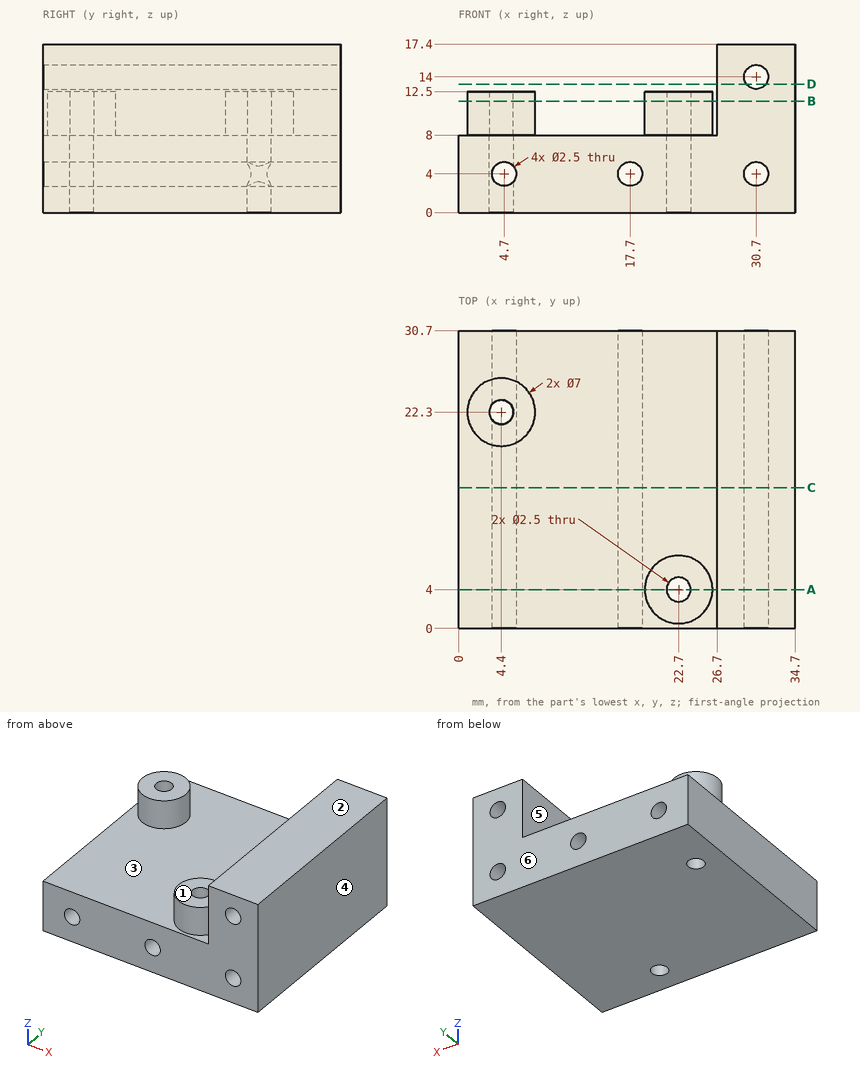
Input: dimensioned drawing with shaded views. Units: mm. Origin: part minimum x, y, z. A direction names the side the tool comes from. Round coordinates to 2 decimals unless told otherwise and drop trailing zeros. Order: outer loops, then holes, each group sorted by start corner. A loop starts at its lowest first (then second) coordinate and runs counter-clockwise, first axis right, second up. Notation, with made-up numbers: (31.25, 28) - (81.25, 28) arc R24 ccw to (81.25, 44) - close; hole circle Ø10 at (1, 70). An arc over 180 degrees is marked (long way). Use CSV: the item, a comma, the result in double quotes. Start each with the question number.
Q1. Section query B-B (z = 11.5). Return loops of the section in (x, y).
Q2. Section query A-A (y = 4). Return loops of the section in (x, z).
Q3. Material intervals for line 1 along X through (y, z) = (21.5, 12); line 2 along X through (y, z) = (13.5, 3.5); line 3 along Z through (x, y) = (19.5, 27.5), sorted ascending. Write a range as from..to.
Q4. Section query C-C (y = 14.5). Return loops of the section in (x, z).
Q5. First-contact query: pin 1 (3 mm diameter, centred on x = 17.7, z = 4, fed in from -Y); pin 2 (2 mm diameter, centred on x = 5.5, y = 22, fed in from +Z); pin 3 (1.5 mm diameter, centred on y = 5, z = 10, fed in from -X); pin 4 (1 mm diameter, centred on x = 19, y = 17, fed in from +Z). Flat tips, straight axial feed; report the tip coordinate or a pass-through.
Q6. Mould query, pull axis X, two halves, no side actions, for the marked faces 4, 5 and 6. Classes: +X half, -X half, draft (parallel to the pull), parting line (faces both ways), or undercut.
Q7. Section query D-D (z = 13.25). Return loops of the section in (x, y), and give its area (3 significant figures).
Q8. Access query for the marked faces 1, 2 and 3. Directions: +Z, -Z, +X, -X, +Y, -Y. A direction counts if a zero-diameter tool reaches every point of the face in a straight line with its end or side. Return the directions, or none.
Result set:
1,outline,"circle Ø7 at (4.4, 22.3); circle Ø7 at (22.7, 4); (26.7, 0) - (34.7, 0) - (34.7, 30.7) - (26.7, 30.7) - close; hole circle Ø2.5 at (4.4, 22.3); hole circle Ø2.5 at (22.7, 4)"
2,outline,"(0, 0) - (21.45, 0) - (21.45, 12.5) - (19.2, 12.5) - (19.2, 8) - (0, 8) - close; (23.95, 0) - (34.7, 0) - (34.7, 17.4) - (26.7, 17.4) - (26.7, 8) - (26.2, 8) - (26.2, 12.5) - (23.95, 12.5) - close; hole circle Ø2.5 at (4.7, 4); hole circle Ø2.5 at (17.7, 4); hole circle Ø2.5 at (30.7, 4); hole circle Ø2.5 at (30.7, 14)"
3,line 1,"x = 0.99..3.44, 5.36..7.81, 26.7..34.7"
3,line 2,"x = 0..3.55, 5.85..16.55, 18.85..29.55, 31.85..34.7"
3,line 3,"z = 0..8"
4,outline,"(0, 0) - (34.7, 0) - (34.7, 17.4) - (26.7, 17.4) - (26.7, 8) - (0, 8) - close; hole circle Ø2.5 at (4.7, 4); hole circle Ø2.5 at (17.7, 4); hole circle Ø2.5 at (30.7, 4); hole circle Ø2.5 at (30.7, 14)"
5,pin 1,"stops at y = 0"
5,pin 2,"stops at z = 12.5"
5,pin 3,"stops at x = 19.21"
5,pin 4,"stops at z = 8"
6,face 4,"+X half"
6,face 5,"undercut"
6,face 6,"draft"
7,outline,"(26.7, 0) - (29.7, 0) - (29.7, 30.7) - (26.7, 30.7) - close; (31.7, 0) - (34.7, 0) - (34.7, 30.7) - (31.7, 30.7) - close"
7,area,"184 mm2"
8,face 1,"+Z, -X, +Y, -Y"
8,face 2,"+Z, +X, -X, +Y, -Y"
8,face 3,"+Z"
